```python
from build123d import *

# Parameters (mm, degrees)
F1_DEPTH = 343.9
F3_D     = 9.525
F4_SIZE  = 10


with BuildPart() as f1:
    # F0 (on Front) → F1 (new body)
    with BuildSketch(Plane.XZ):
        Polygon((0, 76.2), (0, 0), (76.2, 0), (76.2, 5), (5, 5), (5, 76.2), align=None)
    extrude(amount=F1_DEPTH)

    # F3 (through all)
    with Locations(Plane(origin=(0, 0, 0), x_dir=(0, -1, 0), z_dir=(-1, 0, 0))):
        with Locations((127.312, 61.11)):
            Hole(F3_D / 2)

    # F4
    f4_edges = [f1.edges().sort_by_distance(p)[0] for p in [
        (76.2, -343.9, 2.5),
        (2.5, -343.9, 76.2),
    ]]
    chamfer(f4_edges, length=F4_SIZE)


solid = f1.part
```
The model under review builds one solid part; all positions refer to its coordinate system, in mm. A direction names the side the tool comes from. Give positions to 0.01 mm unless a question says otherwise; leave off trailing zeros. Write each loop counter-clockwise with the first axis right and the second up, starting at its lowest first coordinate (ties: lowest second). Pieces come first, ordered by that corner, then holes.
(1) Consider section A-A, the plane z = 61.11. Give the boundary of the cut face in (x, y).
(2) Consider section B-B, the plane y = -55. Give the boundary of the cut face in (x, z), and give its area (3 significant figures).
(3) For P1, Ø4, axis at y = -52.5, z = 37, coming from the +X side; P2, Ø21.5, axis at x = 57, y = -214, coming from the +Z side, all flat-tipped, find the tip position at first contact; note any pin that passes through.
(4) Tool access review of faces 4 (the flat face through (5, -170, 40)), 5 (the flat face through (38, -170, 0)): name each direction out of +Z, -Z, +X, -X, +Y, -Y from which nothing blocks a thin tool from reaching the whole face with its end or side.
(5) To check wall thickness, follow L1, parallel to Y at x = 3, z = 61; L2, parallel to Z at x = 7, y = -107.5. State the ranges of each line that lie inside material, in increasing order.
(6) The part is to be moulded in two halves that separate along Z. For faces 1 (the flat face through (71.3, -338.8, 2.5)), 2 (the flat face through (41, -170, 5)), 3 (the cylindrical face through (2.54, -122.77, 62.54)), say which applies: released by +Z, released by -Z, zero draft, split by the parting line, or undercut.
(7) Consider section C-C, the plane z = 36.5. Give the boundary of the cut face in (x, y), and give its area (3 significant figures).
(8) Consider section D-D, the plane x = 61.5. Give the boundary of the cut face in (y, z).
Returned:
1. outline: (0, -343.9) - (5, -343.9) - (5, -132.07) - (0, -132.07) - close; (0, -122.55) - (5, -122.55) - (5, 0) - (0, 0) - close
2. outline: (0, 0) - (76.2, 0) - (76.2, 5) - (5, 5) - (5, 76.2) - (0, 76.2) - close
2. area: 737 mm2
3. P1: stops at x = 5
3. P2: stops at z = 5
4. face 4: +Z, +X, +Y, -Y
4. face 5: -Z, +X, -X, +Y, -Y
5. L1: y = -343.9 to -132.07, -122.55 to 0
5. L2: z = 0 to 5
6. face 1: zero draft
6. face 2: released by +Z
6. face 3: undercut
7. outline: (0, -343.9) - (5, -343.9) - (5, 0) - (0, 0) - close
7. area: 1,720 mm2
8. outline: (-343.9, 0) - (0, 0) - (0, 5) - (-343.9, 5) - close
